Build history of the part. All positions in model axes, mm. Give positions to 0.01 mm unless a question says otherwise; leave off trailing zeros. Write each loop counter-clockwise with the first axis right and the second up, starting at its lowest first coordinate (ties: lowest second). Pieces come first, ordered by that corner, then holes.
Autodesk Inventor part; units mm, degrees
ref_plane "YZ Plane" through (0, 0, 0) normal (1, 0, 0) x (0, 1, 0)
ref_plane "XZ Plane" through (0, 0, 0) normal (0, 1, 0) x (-1, 0, 0)
ref_plane "XY Plane" through (0, 0, 0) normal (0, 0, 1) x (1, 0, 0)
sketch "Sketch1" plane through (0, 0, 0) normal (0, 0, 1) x (1, 0, 0)
  circle A0 centre (0, 0) radius 16.5
  dimension "d0" = 33
extrude "Extrusion1" add sketch "Sketch1" along normal blind 3
sketch "Sketch2" plane through (0, 0, 3) normal (0, 0, 1) x (1, 0, 0)
  circle A0 centre (0, 0) radius 9 construction
  point P0 (9, 0)
  dimension "d3" = 18
hole "Hole1" at (9, 0, 3) direction (0, 0, -1) diameter 11.6 end through all
pattern_circular "Circular Pattern1" count 3 over 360 about axis through (0, 0, 0) along (0, 0, 1) of "Hole1"
sketch "Sketch3" plane through (0, 0, 3) normal (0, 0, 1) x (1, 0, 0)
  circle A0 centre (0, 0) radius 1.5
  dimension "d14" = 3
extrude "Extrusion2" cut sketch "Sketch3" against normal through all
thread "Thread1"
properties part number "Electrode Aligning Disk" material "Stainless Steel"
1. Drop flat-ended pins along their axis: pin 1 (10 mm diameter, centred on x = 12, y = 0, fed in from -Z); pin 2 (1.5 mm diameter, centred on y = 7.5, z = 0.5, fed in from -X); pin 3 (1 mm diameter, centred on x = -2, y = 4.5, fed in from -Z). Give the stop position or say it passes through.
2. Mould opens along Y. For faces 1 (the face through (-1.5, 0.07, 1.52)), 2 (the face through (3.25, 0.76, 1.48)), 3 (the face through (0, -3, 3)), 4 (the face through (15.24, 6.32, 1.48)) say: pulls with the +Y half, pulls with the -Y half, needs draft (parallel to the pull), parting line crosses it, or undercut.
3. Saw through at B-B on x = 12.5. Give the cut face in (y, z).
4. Saw through at D-D on y = 7.5. Give the cut face in (x, z), plus the area to 3 significant figures.
5. Drill centre lines: line 1 along X through (y, z) = (1, 0.95); line 2 along X through (y, z) = (-5, 2.55); line 3 along Y through (x, z) = (0, 2.1) (3 decimals). Where is each one in solid material? Low to high.
6. Saw through at C-C on x = -4.5. Give the cut face in (y, z), plus the area to 3 significant figures.
7. Saw through at A-A on y = 0. Give the cut face in (x, z), plus the area to 3 significant figures.
Outcome:
1. pin 1: stops at z = 0
1. pin 2: stops at x = -15.06
1. pin 3: passes through
2. face 1: undercut
2. face 2: undercut
2. face 3: needs draft
2. face 4: parting line crosses it
3. outline: (-10.77, 0) - (-4.62, 0) - (-4.62, 3) - (-10.77, 3) - close; (4.62, 0) - (10.77, 0) - (10.77, 3) - (4.62, 3) - close
4. outline: (-14.7, 0) - (-10.29, 0) - (-10.29, 3) - (-14.7, 3) - close; (1.29, 0) - (14.7, 0) - (14.7, 3) - (1.29, 3) - close
4. area: 53.4 mm2
5. line 1: x = -16.47 to -1.12, 1.12 to 3.29, 14.71 to 16.47
5. line 2: x = -15.72 to -9.58, 0.58 to 6.06, 11.94 to 15.72
5. line 3: y = -16.5 to -11.453, -4.135 to -1.5, 1.5 to 4.135, 11.453 to 16.5
6. outline: (-15.87, 0) - (-13.59, 0) - (-13.59, 3) - (-15.87, 3) - close; (-1.99, 0) - (1.99, 0) - (1.99, 3) - (-1.99, 3) - close; (13.59, 0) - (15.87, 0) - (15.87, 3) - (13.59, 3) - close
6. area: 25.6 mm2
7. outline: (-16.5, 0) - (-1.5, 0) - (-1.5, 3) - (-16.5, 3) - close; (1.5, 0) - (3.2, 0) - (3.2, 3) - (1.5, 3) - close; (14.8, 0) - (16.5, 0) - (16.5, 3) - (14.8, 3) - close
7. area: 55.2 mm2
